```python
from build123d import *

# Parameters (mm, degrees)
MODEL_R             = 4
MODEL_R_2           = 7.5
MODEL_W             = 10
MODEL_H             = 12.4
BOSS_EXTRUDE1_DEPTH = 12.4


with BuildPart() as part:
    # Model → Boss-Extrude1 (new body)
    with BuildSketch(Plane.XY):
        Polygon((-12.5, 0), (-15, 2.5), (-15, 131.5), (-12.5, 134), (15, 134), (15, 114), (27.4, 114), (27.4, 84), (15, 84), (15, 50), (27.4, 50), (27.4, 20), (15, 20), (15, 0), align=None)
        with Locations(Location((0, 50.609916554, 0), (0, 0, 180))):
            Circle(MODEL_R, mode=Mode.SUBTRACT)
        with Locations(Location((0, 83.390083446, 0), (0, 0, 180))):
            Circle(MODEL_R, mode=Mode.SUBTRACT)
        with Locations(Location((0, 15, 0), (0, 0, 180))):
            Circle(MODEL_R_2, mode=Mode.SUBTRACT)
        with Locations(Location((0, 119, 0), (0, 0, 180))):
            Circle(MODEL_R_2, mode=Mode.SUBTRACT)
        with Locations((0, 99)):
            Rectangle(MODEL_W, MODEL_H, mode=Mode.SUBTRACT)
        Polygon((0, 74.390083446), (-6.4, 70.695041723), (-6.4, 63.304958277), (0, 59.609916554), (6.4, 63.304958277), (6.4, 70.695041723), align=None, mode=Mode.SUBTRACT)
        with Locations((0, 35)):
            Rectangle(MODEL_W, MODEL_H, mode=Mode.SUBTRACT)
    extrude(amount=BOSS_EXTRUDE1_DEPTH)


solid = part.part
```
The model under review builds one solid part; all positions refer to its coordinate system, in mm. A direction names the side the tool comes from. Round coordinates to 2 decimals unless told otherwise and drop trailing zeros. Write each loop counter-clockwise with the first axis right and the second up, starting at its lowest first coordinate (ties: lowest second). Pieces come first, ordered by that corner, then holes. Notation, with made-up numbers: (22, -2) - (61, -2) arc R13 cw to (61, 3) - close; hole circle Ø1 at (74, 40.5). An arc over 180 degrees is marked (long way). Answer as CSV lines item,"result". Start each with the question number.
(1) To check wall thickness, follow line 1 (X direction, y = 119, z = 4.25); line 2 (X direction, y = 67, z = 0.75); line 3 (Y direction, x = 25.5, z = 11). State the ranges of each line that lie inside material, in increasing order.
(2) We need section A-A on y = 100. State the section outline as (x, z) points, plus the area to 3 significant figures.
(3) For faces 1 (the flat face through (-13.8, 132.7, 6.1)), 2 (the flat face through (-3.155, 72.568, 6.113)), 3 (the flat face through (15, 67, 6)), 4 (the flat face through (15, 10, 6)), 5 (the flat face through (15, 124, 6)), list the 3-axis set-ups (+Z, -Z, +X, -X, +Y, -Y) from which the entire face can be reached by the end or side of a thin tool; tool diameter is ignored.
(4) We need section C-C on y = 119. State the section outline as (x, z) points, plus the area to 3 significant figures.
(5) We need section D-D on y = 77. State the section outline as (x, z) points.
(6) For pin 1 Ø3.5 at (y, z) = (120.5, 5) entering from +X, flat-tipped, find the tip position at first contact; note if it passes through.
(7) Draft analysis for pull direction X (two halves, no side actions). For faces 6 (the flat face through (-5, 99, 6)), 7 (the flat face through (21, 114, 6)), 8 (the cylindrical face through (1.63, 126.32, 6.11)), 9 (the flat face through (-13.7, 1.2, 6.1)), state which applies: pulls with the +X half, pulls with the -X half, needs draft (parallel to the pull), parting line crosses it, or undercut.
(8) We need section B-B on z = 7.5. Give the number of separate pieces and of enclosed holes in the cut face, plus the area to 3 significant figures.
Worked answers:
1,line 1,"-15 to -7.5, 7.5 to 15"
1,line 2,"-15 to -6.4, 6.4 to 15"
1,line 3,"20 to 50, 84 to 114"
2,outline,"(-15, 0) - (-5, 0) - (-5, 12.4) - (-15, 12.4) - close; (5, 0) - (27.4, 0) - (27.4, 12.4) - (5, 12.4) - close"
2,area,"402 mm²"
3,face 1,"+Z, -Z, -X, +Y"
3,face 2,"+Z, -Z"
3,face 3,"+Z, -Z, +X"
3,face 4,"+Z, -Z, +X, -Y"
3,face 5,"+Z, -Z, +X, +Y"
4,outline,"(-15, 0) - (-7.5, 0) - (-7.5, 12.4) - (-15, 12.4) - close; (7.5, 0) - (15, 0) - (15, 12.4) - (7.5, 12.4) - close"
4,area,"186 mm²"
5,outline,"(-15, 0) - (15, 0) - (15, 12.4) - (-15, 12.4) - close"
6,pin 1,"x = 15"
7,face 6,"undercut"
7,face 7,"needs draft"
7,face 8,"undercut"
7,face 9,"pulls with the -X half"
8,separate pieces,"1"
8,enclosed holes,"7"
8,area,"3,910 mm²"
